```python
from build123d import *

# Parameters (mm, degrees)
F2_W     = 0.5
F2_H     = 2
F3_DEPTH = 79
F4_DEPTH = 77
F5_SIZE  = 0.49999


# Not quite as in the source:
# - a fillet or chamfer is up to 0.001 mm smaller than in the source, because OpenCascade refuses the exact size


with BuildPart() as f3:
    # F2 (on Front) → F3 (new body, symmetric)
    with BuildSketch(Plane.XZ):
        with BuildLine():
            Line((-27, -19), (-27, -17))
            Line((-27, -17), (-27.5, -17))
            Line((-27.5, -17), (-27.5, -15))
            Line((-27.5, -15), (-27.5, -13))
            Line((-27.5, -13), (-27.5, 13))
            Line((-27.5, 13), (-27.5, 15))
            Line((-27.5, 15), (-27, 15))
            Line((-27, 15), (-25.5, 15))
            Line((-25.5, 15), (0, 15))
            Line((0, 15), (25.5, 15))
            Line((25.5, 15), (27, 15))
            Line((27, 15), (27.5, 15))
            Line((27.5, 15), (27.5, 13))
            Line((27.5, 13), (27.5, -13))
            Line((27.5, -13), (27.5, -15))
            Line((27.5, -15), (27.5, -17))
            Line((27.5, -17), (27, -17))
            Line((27, -17), (27, -19))
            Line((27, -19), (31, -19))
            Line((31, -19), (31, 15))
            ThreePointArc((31, 15), (30.4142135624, 16.4142135624), (29, 17))
            Line((29, 17), (0, 17))
            Line((0, 17), (-29, 17))
            ThreePointArc((-29, 17), (-30.4142135624, 16.4142135624), (-31, 15))
            Line((-31, 15), (-31, -19))
            Line((-31, -19), (-27, -19))
        make_face()
        with Locations((-27.25, -14)):
            Rectangle(F2_W, F2_H)
        with BuildLine():
            Line((-27.5, 13), (-27.5, -13))
            Line((-27.5, -13), (-27, -13))
            Line((-27, -13), (-27, 14.3228756555))
            ThreePointArc((-27, 14.3228756555), (-27.3708286934, 13.7071067812), (-27.5, 13))
        make_face()
        with BuildLine():
            Line((-27.5, 15), (-27.5, 13))
            ThreePointArc((-27.5, 13), (-27.3708286934, 13.7071067812), (-27, 14.3228756555))
            Line((-27, 14.3228756555), (-27, 15))
            Line((-27, 15), (-27.5, 15))
        make_face()
        with BuildLine():
            Line((-27, 15), (-27, 14.3228756555))
            ThreePointArc((-27, 14.3228756555), (-26.3228756555, 14.8228756555), (-25.5, 15))
            Line((-25.5, 15), (-27, 15))
        make_face()
        with BuildLine():
            Line((27, 15), (25.5, 15))
            ThreePointArc((25.5, 15), (26.3228756555, 14.8228756555), (27, 14.3228756555))
            Line((27, 14.3228756555), (27, 15))
        make_face()
        with BuildLine():
            Line((27.5, 15), (27, 15))
            Line((27, 15), (27, 14.3228756555))
            ThreePointArc((27, 14.3228756555), (27.3708286934, 13.7071067812), (27.5, 13))
            Line((27.5, 13), (27.5, 15))
        make_face()
        with BuildLine():
            ThreePointArc((27.5, 13), (27.3708286934, 13.7071067812), (27, 14.3228756555))
            Line((27, 14.3228756555), (27, -13))
            Line((27, -13), (27.5, -13))
            Line((27.5, -13), (27.5, 13))
        make_face()
        with Locations((27.25, -14)):
            Rectangle(F2_W, F2_H)
    extrude(amount=F3_DEPTH, both=True)

    # F2 (on Front) → F4 (cut, symmetric)
    with BuildSketch(Plane.XZ):
        with BuildLine():
            Line((-27.5, 13), (-27.5, -13))
            Line((-27.5, -13), (-27, -13))
            Line((-27, -13), (-27, 14.3228756555))
            ThreePointArc((-27, 14.3228756555), (-27.3708286934, 13.7071067812), (-27.5, 13))
        make_face()
        with BuildLine():
            Line((-27.5, 15), (-27.5, 13))
            ThreePointArc((-27.5, 13), (-27.3708286934, 13.7071067812), (-27, 14.3228756555))
            Line((-27, 14.3228756555), (-27, 15))
            Line((-27, 15), (-27.5, 15))
        make_face()
        with BuildLine():
            ThreePointArc((27.5, 13), (27.3708286934, 13.7071067812), (27, 14.3228756555))
            Line((27, 14.3228756555), (27, -13))
            Line((27, -13), (27.5, -13))
            Line((27.5, -13), (27.5, 13))
        make_face()
    extrude(amount=F4_DEPTH, both=True, mode=Mode.SUBTRACT)

    # F5 (size 0.5 in the source; OpenCascade refuses exactly that, so slightly less here)
    f5_edges = [f3.edges().sort_by_distance(p)[0] for p in [
        (-27, 0, -17),
        (-27, 0, -15),
        (27, 0, -15),
        (27, 0, -17),
        (-27, 0, -19),
        (27, 0, -19),
        (-31, 0, -19),
        (31, 0, -19),
    ]]
    chamfer(f5_edges, length=F5_SIZE)


solid = f3.part
```
Geometry: final body of the model. Coordinates: model frame, mm. A direction names the side the tool comes from. Round coordinates to 2 decimals unless told otherwise and drop trailing zeros. Order: outer loops, then holes, each group sorted by start corner. A loop starts at its lowest first (then second) coordinate and runs counter-clockwise, first axis right, second up. Notation, with made-up numbers: (86.25, -32.5) - (114.25, -32.5) arc R23 ccw to (114.25, -14.5) - close; hole circle Ø1 at (54.5, 84). An arc over 180 degrees is marked (long way). Write item = value, one per line. Start each with the question number.
Q1. Cut plane B-B on x = 7. Return the cut outline in (y, z), and give its area (3 significant figures).
Q2. Ray query, line 1 (X direction, y = -41.5, z = -9); line 2 (X direction, y = 5.5, z = -14); line 3 (Z direction, x = 20, y = 31). Return the intervals inside material, ascending. Write a range as from..to.
Q3. Cut plane A-A on z = -4.5. Return the cut outline in (x, y), and give its area (3 significant figures).
Q4. Pin query (flat end, axial travel): pin 1 (15.5 mm diameter, centred on x = 12, y = 2.5, fed in from -Z). Return the tip coordinate at first contact, or that it passes through.
Q5. Pull-direction query (X, two-part tool) for faces 1 (the flat face through (0, -1, 17)), 2 (the flat face through (27, 0, -14)), 3 (the flat face through (31, -1, -2)), 4 (the flat face through (27.5, -1, 0)); classes: +X half, -X half, draft (parallel to the pull), parting line (faces both ways), or undercut.
Q6. Access query for faces 5 (the flat face through (-31, -1, -2)), 6 (the flat face through (-27.5, 1, 1)), 7 (the flat face through (0, -1, 15)). Directions: +Z, -Z, +X, -X, +Y, -Y. A direction counts if a zero-diameter tool reaches every point of the face in a straight line with its end or side. Return the directions, or none.
Outcome:
q1.outline = (-79, 15) - (79, 15) - (79, 17) - (-79, 17) - close
q1.area = 316 mm^2
q2.line_1 = -31..-27.5, 27.5..31
q2.line_2 = -31..-27, 27..31
q2.line_3 = 15..17
q3.outline = (-31, -79) - (-27, -79) - (-27, -77) - (-27.5, -77) - (-27.5, 77) - (-27, 77) - (-27, 79) - (-31, 79) - close; (27, -79) - (31, -79) - (31, 79) - (27, 79) - (27, 77) - (27.5, 77) - (27.5, -77) - (27, -77) - close
q3.area = 1,110 mm^2
q4.pin_1 = 15
q5.face_1 = draft
q5.face_2 = undercut
q5.face_3 = +X half
q5.face_4 = undercut
q6.face_5 = +Z, -Z, -X, +Y, -Y
q6.face_6 = none
q6.face_7 = -Z, +Y, -Y
